```python
from build123d import *

# Parameters (mm, degrees)
F1_DEPTH = 36.5125
F2_R     = 2.0193
F3_DEPTH = 4.7625
F4_R     = 3.17499


# Not quite as in the source:
# - a fillet or chamfer is up to 0.001 mm smaller than in the source, because OpenCascade refuses the exact size


with BuildPart() as f1:
    # F0 (on Right) → F1 (new body)
    with BuildSketch(Plane.YZ):
        Polygon((-4.7625, 0), (0, 0), (0, 31.75), (-4.7625, 31.75), (-4.7625, 19.05), (-10.2997, 19.05), (-10.2997, 12.7), (-4.7625, 12.7), align=None)
    extrude(amount=-F1_DEPTH)

    # F2 (on face) → F3 (cut, through all)
    with BuildSketch(Plane.XZ.offset(4.7625)):
        with Locations((-18.25625, 25.019)):
            Circle(F2_R)
        with Locations((-18.25625, 6.731)):
            Circle(F2_R)
    extrude(amount=-F3_DEPTH, mode=Mode.SUBTRACT)

    # F4 (radius 3.175 in the source; OpenCascade refuses exactly that, so slightly less here)
    f4_edges = [f1.edges().sort_by_distance(p)[0] for p in [
        (0, -7.5311, 19.05),
        (0, -7.5311, 12.7),
        (-36.5125, -7.5311, 12.7),
        (-36.5125, -7.5311, 19.05),
    ]]
    fillet(f4_edges, radius=F4_R)


solid = f1.part
```
The listing builds one solid part. Answer for the finished solid, in the listing's coordinates (mm). A direction names the side the tool comes from. Coordinates: 2 decimals unless noted, no trailing zeros. Order: outer loops, then holes, each group sorted by start corner. A loop starts at its lowest first (then second) coordinate and runs counter-clockwise, first axis right, second up. Notation, with made-up numbers: M 71,7.25 L 129,7.25 A19 ccw 129,38.25 Z; hole C 82,18 d11. An arc over 180 degrees is marked long. Answer as a JSON object with one key per item and string values. Group by question number.
1. A tool of negligible diameter and unlimited length cuts with its end or side. For faces 4 (the cylindrical face through (-35.607, -7.492, 13.655)), 5 (the cylindrical face through (-0.91, -7.57, 18.1)), 6 (the cylindrical face through (-0.91, -7.49, 13.65)), from which of +Z, -Z, +X, -X, +Y, -Y can it reach the whole face along a straight path? Write none if from no direction.
2. Flat-ended cylindrical pins translate along their axes: P1, Ø5.5, axis at x = -18.26, z = 25.02, coming from the -Y side; P2, Ø12.5, axis at x = -23.5, z = 20, coming from the -Y side; P3, Ø6, axis at y = -9, z = 21.5, coming from the -X side; P4, Ø1.5, axis at x = -32, y = -6, coming from the -Z side. Find the tip coordinate at first contact, or state that the pin passes through.
3. Section C-C on x = -14 is taken. Write down the section's boundary in (y, z), then the cut area to 3 significant figures.
4. Section D-D on y = -2.5 is taken. Write down the section's boundary in (x, z), then the cut area to 3 significant figures.
5. Section B-B on z = 8 is taken. Write down the section's boundary in (x, y), then the cut area to 3 significant figures.
6. Determine the mould class of faces 1 (the cylindrical face through (-18.694, -2.415, 23.048)), 2 (the flat face through (-36.512, -3, 16)), 3 (the flat face through (-18, -8, 12.7)) for opening direction Z: released by +Z, released by -Z, zero draft, split by the parting line, or undercut.
7. Straight lines are drawn through the part: line 1 (Y direction, x = -26, z = 4); line 2 (X direction, y = -0.75, z = 24); line 3 (X direction, y = -0.25, z = 8). For each, find the intervals that lie inside material, in ascending order.
Values follow:
{
 "1": {"face 4": "-Z, -X, -Y", "face 5": "+Z, +X, -Y", "face 6": "-Z, +X, -Y"},
 "2": {"P1": "y = -4.76", "P2": "y = -10.3", "P3": "x = -35.12", "P4": "z = 12.7"},
 "3": {"outline": "M -10.3,12.7 L -4.76,12.7 L -4.76,0 L 0,0 L 0,31.75 L -4.76,31.75 L -4.76,19.05 L -10.3,19.05 Z", "area": "186 mm2"},
 "4": {"outline": "M -36.51,0 L 0,0 L 0,31.75 L -36.51,31.75 Z; hole C -18.26,6.73 d4.04; hole C -18.26,25.02 d4.04", "area": "1,130 mm2"},
 "5": {"outline": "M -36.51,-4.76 L -19.83,-4.76 L -19.83,0 L -36.51,0 Z; M -16.69,-4.76 L 0,-4.76 L 0,0 L -16.69,0 Z", "area": "159 mm2"},
 "6": {"face 1": "undercut", "face 2": "zero draft", "face 3": "released by -Z"},
 "7": {"line 1": "-4.76 to 0", "line 2": "-36.51 to -20, -16.51 to 0", "line 3": "-36.51 to -19.83, -16.69 to 0"}
}
